The model under review builds one solid part; all positions refer to its coordinate system, in mm. A direction names the side the tool comes from. Coordinates: 2 decimals unless noted, no trailing zeros. Order: outer loops, then holes, each group sorted by start corner. A loop starts at its lowest first (then second) coordinate and runs counter-clockwise, first axis right, second up. Notation, with made-up numbers: M -13,-36 L 31,-36 A25 ccw 31,-6 Z; hole C 54,87.25 d6. An arc over 180 degrees is marked long. Answer in a Markdown table with one row per item.
from build123d import *

# Parameters (mm, degrees)
SKETCH1_R               = 2.25
SKETCH1_R_2             = 4.15
SKETCH1_R_3             = 4.09
SKETCH1_R_4             = 1.6
SKETCH1_W               = 42.14
SKETCH1_H               = 42.14
SALIENTE_EXTRUIR1_DEPTH = 27
REDONDEO1_R             = 42.5
REDONDEO2_R             = 10
CORTAR_EXTRUIR1_DEPTH   = 10.2
CORTAR_EXTRUIR2_DEPTH   = 3.39


with BuildPart() as part:
    # Sketch1 → Saliente-Extruir1 (new body)
    with BuildSketch(Plane(origin=(0, 0, 0), x_dir=(1, 0, 0), z_dir=(0, 1, 0))):
        with BuildLine():
            ThreePointArc((0, 60), (-60, 0), (0, -60))
            ThreePointArc((0, -60), (23.048861143, -57.469875145), (45, -50))
            ThreePointArc((45, -50), (119.487995331, -32.139859918), (195, -45))
            ThreePointArc((195, -45), (240, 0), (195, 45))
            ThreePointArc((195, 45), (119.487995331, 32.139859918), (45, 50))
            ThreePointArc((45, 50), (23.048861143, 57.469875145), (0, 60))
        make_face()
        with Locations(Location((-20, -20, 0), (0, 0, 270))):
            Circle(SKETCH1_R, mode=Mode.SUBTRACT)
        with Locations(Location((20, -20, 0), (0, 0, 270))):
            Circle(SKETCH1_R, mode=Mode.SUBTRACT)
        with Locations(Location((-20, 20, 0), (0, 0, 270))):
            Circle(SKETCH1_R, mode=Mode.SUBTRACT)
        with Locations(Location((20, 20, 0), (0, 0, 270))):
            Circle(SKETCH1_R, mode=Mode.SUBTRACT)
        with Locations(Location((0, 0, 0), (0, 0, 270))):
            Circle(SKETCH1_R_2, mode=Mode.SUBTRACT)
        with Locations(Location((195, 0, 0), (0, 0, 270))):
            Circle(SKETCH1_R_3, mode=Mode.SUBTRACT)
        with Locations(Location((195, -15, 0), (0, 0, 270))):
            Circle(SKETCH1_R_4, mode=Mode.SUBTRACT)
        with Locations(Location((195, 15, 0), (0, 0, 270))):
            Circle(SKETCH1_R_4, mode=Mode.SUBTRACT)
        with Locations((114.74, 0)):
            Rectangle(SKETCH1_W, SKETCH1_H, mode=Mode.SUBTRACT)
    extrude(amount=SALIENTE_EXTRUIR1_DEPTH)

    # Redondeo1
    # the kernel refuses this fillet: 42.5 mm, written as the material it takes off along each edge
    with BuildSketch(Plane(origin=(195, -132.493054203, -45), x_dir=(0.8082364962283539, 0, 0.5888580186806613), z_dir=(0, 1, 0))) as redondeo1_piece_1:
        with BuildLine():
            CenterArc((27.970755887, -34.35005109), REDONDEO1_R, 53.923988444, 90)
            ThreePointArc((-6.379295202, -9.323585296), (-3.120659761, -4.708994854), (0, 0))
            ThreePointArc((0, 0), (26.498610841, 8.62935767), (52.997221681, 0))
        make_face()
    extrude(amount=291.986108406, mode=Mode.SUBTRACT)
    with BuildSketch(Plane(origin=(195, -132.493054203, 45), x_dir=(-0.9423869480769151, 0, -0.3345247974280495), z_dir=(0, 1, 0))) as redondeo1_piece_2:
        with BuildLine():
            CenterArc((12.554710632, -42.481389287), REDONDEO1_R, 91.695666833, 90)
            ThreePointArc((-29.926678654, -43.73899188), (-22.085210872, -16.996636462), (0, 0))
            ThreePointArc((0, 0), (5.64855402, -0.083590492), (11.297108039, 0))
        make_face()
    extrude(amount=291.986108406, mode=Mode.SUBTRACT)

    # Redondeo2
    redondeo2_edges = [part.edges().sort_by_distance(p)[0] for p in [
        (23.048861143, 27, 57.469875145),
        (113.845361587, 27, 32.411584628),
        (23.048861143, 27, -57.469875145),
        (240, 0, 0),
        (240, 27, 0),
        (113.845361587, 0, -32.411584628),
        (216.774685632, 0, -38.582680786),
        (216.774685632, 0, 38.582680786),
        (113.845361587, 27, -32.411584628),
        (216.774685632, 27, -38.582680786),
        (216.774685632, 27, 38.582680786),
        (113.845361587, 0, 32.411584628),
        (23.048861143, 0, 57.469875145),
        (-60, 0, 0),
        (23.048861143, 0, -57.469875145),
        (-60, 27, 0),
    ]]
    fillet(redondeo2_edges, radius=REDONDEO2_R)

    # Croquis1 → Cortar-Extruir1 (cut)
    with BuildSketch(Plane.XZ):
        with BuildLine():
            Line((207.7, 17.4), (207.7, -17.4))
            ThreePointArc((207.7, -17.4), (195, -30.1), (182.3, -17.4))
            Line((182.3, -17.4), (182.3, 17.4))
            ThreePointArc((182.3, 17.4), (195, 30.1), (207.7, 17.4))
        make_face()
    extrude(amount=-CORTAR_EXTRUIR1_DEPTH, mode=Mode.SUBTRACT)

    # Croquis2 → Cortar-Extruir2 (cut)
    with BuildSketch(Plane(origin=(0, 27, 0), x_dir=(1, 0, 0), z_dir=(0, 1, 0))):
        Polygon((199.110733917, 15), (197.055366958, 18.56), (192.944633042, 18.56), (190.889266083, 15), (192.944633042, 11.44), (197.055366958, 11.44), align=None)
        Polygon((197.055366958, -11.44), (192.944633042, -11.44), (190.889266083, -15), (192.944633042, -18.56), (197.055366958, -18.56), (199.110733917, -15), align=None)
    extrude(amount=-CORTAR_EXTRUIR2_DEPTH, mode=Mode.SUBTRACT)


solid = part.part
(1) The part is to be moulded in two halves that separate along X. For faces 4 (the cylindrical face through (23.37, 13.45, -57.4)), 5 (the cylindrical face through (112.847, 13.451, 32.477)), 6 (the flat face through (57, 0, -1)), say which applies: +X half, -X half, draft (parallel to the pull), parting line (faces both ways), or undercut.
Report:
| item | result |
|---|---|
| face 4 | +X half |
| face 5 | undercut |
| face 6 | draft |
(2) To check wall thickness, follow line 1 (X direction, y = 17.5, z = 0); line 2 (X direction, y = 21.5, z = -20); line 3 (Z direction, x = 195, y = 15.75). State the ranges of each line that lie inside material, in increasing order. Write a range as [from, to].
Report:
| item | result |
|---|---|
| line 1 | [-59.99, -4.15], [4.15, 93.67], [135.81, 190.91], [199.09, 239.99] |
| line 2 | [-55.43, -22.25], [-17.75, 17.75], [22.25, 93.67], [135.81, 234.07] |
| line 3 | [-43.2, -16.6], [-13.4, -4.09], [4.09, 13.4], [16.6, 43.2] |
(3) Take a section at B-B (y = 2.75). Write out the cut boundary in (x, z), then the cut area to 3 significant figures.
Report:
| item | result |
|---|---|
| outline | M 0,-56.89 A103.14 ccw 43.68,-47.18 A194 cw 185.31,-38.26 A39.39 ccw 234.87,-12.84 A41.89 ccw 234.87,12.84 A39.39 ccw 185.31,38.26 A194 cw 43.68,47.18 A103.14 ccw 0,56.89 A56.89 ccw Z; hole C -20,-20 d4.5; hole C -20,20 d4.5; hole C 0,0 d8.3; hole C 20,-20 d4.5; hole C 20,20 d4.5; hole M 93.67,-21.07 L 135.81,-21.07 L 135.81,21.07 L 93.67,21.07 Z; hole M 182.3,-17.4 A12.7 ccw 207.7,-17.4 L 207.7,17.4 A12.7 ccw 182.3,17.4 Z |
| area | 19,500 mm^2 |
(4) Machinability: for faces 1 (the cylindrical face through (195.279, 5.029, -30.097)), 2 (the flat face through (93.67, 13, 0)), 3 (the cylindrical face through (240, 13, 0)), which of the approach directions +Z, -Z, +X, -X, +Y, -Y give a long, thin tool a straight path to every point of the face, cutting with its end or side? Answer none if there is none.
Report:
| item | result |
|---|---|
| face 1 | -Y |
| face 2 | +Y, -Y |
| face 3 | +X, +Y, -Y |
(5) Take a section at A-A (z = 0). Write out the cut boundary in (x, y), then the cut area to 3 significant figures.
Report:
| item | result |
|---|---|
| outline | M -60,10 A10 ccw -50,0 L -4.15,0 L -4.15,27 L -50,27 A10 ccw -60,17 Z; M 4.15,0 L 93.67,0 L 93.67,27 L 4.15,27 Z; M 135.81,0 L 182.3,0 L 182.3,10.2 L 190.91,10.2 L 190.91,27 L 135.81,27 Z; M 199.09,10.2 L 207.7,10.2 L 207.7,0 L 230,0 A10 ccw 240,10 L 240,17 A10 ccw 230,27 L 199.09,27 Z |
| area | 6,260 mm^2 |
(6) Insertion check: P1, Ø3, axis at y = 8.5, z = 37, coming from the -X side; P2, Ø1, axis at x = 70.5, y = 13.5, coming from the -Z side; P3, Ø1.7, axis at x = 194.5, y = 25, coming from the +Z side; P4, Ø4, axis at x = 4, z = -27, coming from the -Y side. Each pin has a flat end and moves straight along its axis. Give the tip position at first contact, or say it passes through.
Report:
| item | result |
|---|---|
| P1 | x = -48.26 |
| P2 | z = -40.39 |
| P3 | z = 40.15 |
| P4 | y = 0 |
